Input: dimensioned drawing with shaded views. Units: mm. Origin: part minimum x, y, z. A direction names the side the tool comes from. Round coordinates to 2 decimals unless told otherwise and drop trailing zeros. Loops run counter-clockwise (first coordinate to the right, second up) from the corner with the lowest first, then second, coordinate; pieces in that order, holes last. Notation, with made-up numbers: M -38.5,49.25 L -11.5,49.25 A30 ccw -11.5,71.25 Z; hole C -16,-35 d10. An arc over 180 degrees is marked long. Answer as a JSON object with one key per item and string values.
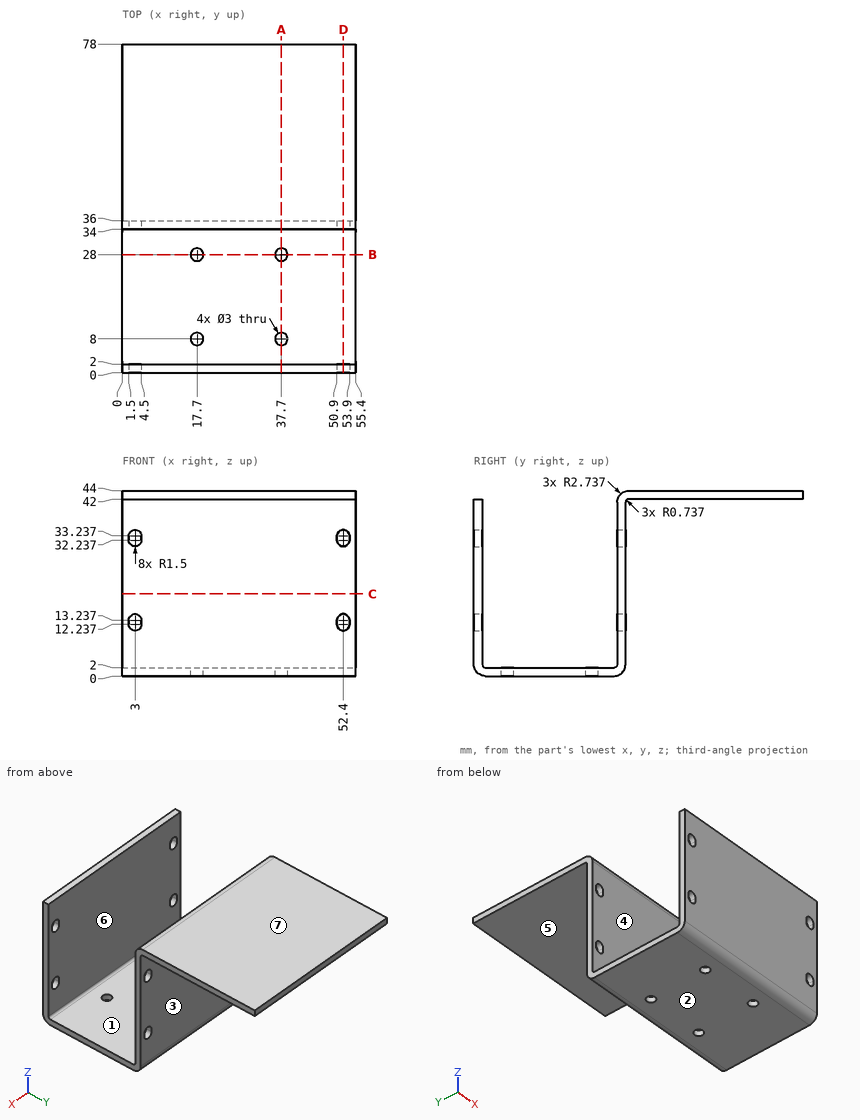
Item 1: Pull-direction query (Y, two-part tool) for the marked faces 1, 2, 3 and 4; classes: pulls with the +Y half, pulls with the -Y half, needs draft (parallel to the pull), parting line crosses it, or undercut.
Answer sheet:
{"face 1": "undercut", "face 2": "needs draft", "face 3": "pulls with the +Y half", "face 4": "undercut"}
Item 2: Section C-C on z = 19.5. Return the cut outline in (x, y).
Answer sheet:
{"outline": "M 0,0 L 55.4,0 L 55.4,2 L 0,2 Z; M 0,34 L 55.4,34 L 55.4,36 L 0,36 Z"}
Item 3: Section B-B on y = 28. Return the cut outline in (x, z).
Answer sheet:
{"outline": "M 0,0 L 16.2,0 L 16.2,2 L 0,2 Z; M 19.2,0 L 36.2,0 L 36.2,2 L 19.2,2 Z; M 39.2,0 L 55.4,0 L 55.4,2 L 39.2,2 Z"}
Item 4: Contact query for flat-ended pins moving along their axis: pin 1 Ø2 at (y, z) = (33.5, 15) entering from +X; pin 2 Ø1 at (x, y) = (15, 0.5) entering from +Z; pin 3 Ø5 at (x, z) = (10, 10.5) entering from +Y; pin 4 Ø10 at (y, z) = (24.5, 16.5) entering from +X. Output: stop coordinate, or through.
Answer sheet:
{"pin 1": "stops at x = 55.4", "pin 2": "stops at z = 42", "pin 3": "stops at y = 36", "pin 4": "passes through"}
Item 5: Section D-D on x = 52.4. Give the number of separate pieces and of enclosed holes in the cut face.
Answer sheet:
{"separate pieces": "5", "enclosed holes": "0"}
Item 6: Line query: probe 1 along Y at (x, z) = (17.7, 1.3); probe 2 along Y at (x, z) = (37, 1) (1 decimal); probe 3 along Y at (x, z) = (52.5, 15.5). Output: solid intervals per line, ascending. Write a range as from..to.
Answer sheet:
{"probe 1": "y = 0.41..6.5, 9.5..26.5, 29.5..35.59", "probe 2": "y = 0.6..6.7, 9.3..26.7, 29.3..35.4", "probe 3": "y = 0..2, 34..36"}
Item 7: Section A-A on x = 37.7. Return the cut outline in (y, z).
Answer sheet:
{"outline": "M 0,2.74 A2.74 ccw 2.74,0 L 6.5,0 L 6.5,2 L 2.74,2 A0.74 cw 2,2.74 L 2,42 L 0,42 Z; M 9.5,0 L 26.5,0 L 26.5,2 L 9.5,2 Z; M 29.5,0 L 33.26,0 A2.74 ccw 36,2.74 L 36,41.26 A0.74 cw 36.74,42 L 78,42 L 78,44 L 36.74,44 A2.74 ccw 34,41.26 L 34,2.74 A0.74 cw 33.26,2 L 29.5,2 Z"}
Item 8: Access query for the marked faces 5, 6 and 7. Directions: +Z, -Z, +X, -X, +Y, -Y. A direction counts if a zero-diameter tool reaches every point of the face in a straight line with its end or side. Return the directions, or none.
Answer sheet:
{"face 5": "-Z, +X, -X, +Y", "face 6": "+Z, +X, -X", "face 7": "+Z, +X, -X, +Y, -Y"}
